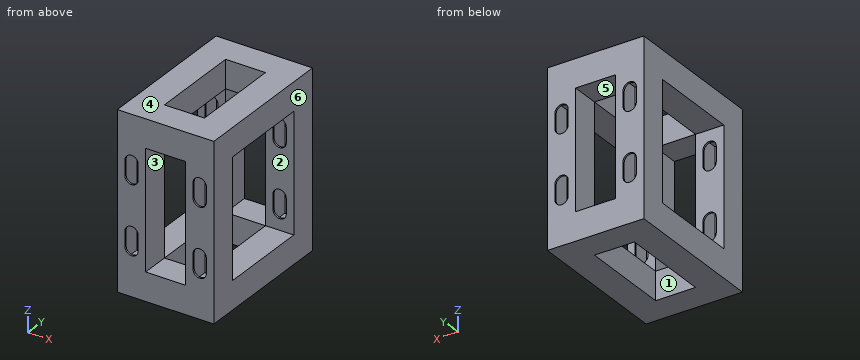
```python
from build123d import *

# Parameters (mm, degrees)
SKETCH2_W          = 19.05
SKETCH2_H          = 19.05
SKETCH2_W_2        = 16.65
SKETCH2_H_2        = 16.65
CUT_EXTRUDE1_START = -9.525
SKETCH1_3_W        = 26.96
SKETCH1_3_H        = 80
CUT_EXTRUDE1_DEPTH = 19.05
SKETCH4_W          = 19.05
SKETCH4_H          = 19.05
SKETCH4_W_2        = 16.65
SKETCH4_H_2        = 16.65


with BuildPart() as part:
    # Sweep1: sweep along a path in Sketch1
    with BuildLine(Plane(origin=(0, 0, 0), x_dir=(1, 0, 0), z_dir=(0, 1, 0))) as sweep1_path:
        Line((13.48, 40), (-13.48, 40))
        Line((-13.48, 40), (-13.48, -40))
        Line((-13.48, -40), (13.48, -40))
        Line((13.48, -40), (13.48, 40))
    # Sketch2 → Sweep1 (sweep)
    with BuildSketch(Plane.XY):
        with Locations((-23.005, 0)):
            Rectangle(SKETCH2_W, SKETCH2_H)
        with Locations((-23.005, 0)):
            Rectangle(SKETCH2_W_2, SKETCH2_H_2, mode=Mode.SUBTRACT)
    sweep(path=sweep1_path.line, transition=Transition.RIGHT)

    # Sketch1<3> → Cut-Extrude1 (cut)
    with BuildSketch(Plane(origin=(0, 0, 0), x_dir=(1, 0, 0), z_dir=(0, 1, 0)).offset(CUT_EXTRUDE1_START)):
        Rectangle(SKETCH1_3_W, SKETCH1_3_H)
        with BuildLine():
            Line((-18.480970389, 27.980970389), (-18.480970389, 17.980970389))
            ThreePointArc((-18.480970389, 17.980970389), (-22.980970389, 13.480970389), (-27.480970389, 17.980970389))
            Line((-27.480970389, 17.980970389), (-27.480970389, 27.980970389))
            ThreePointArc((-27.480970389, 27.980970389), (-22.980970389, 32.480970389), (-18.480970389, 27.980970389))
        make_face()
        with BuildLine():
            Line((-18.480970389, -17.980970389), (-18.480970389, -27.980970389))
            ThreePointArc((-18.480970389, -27.980970389), (-22.980970389, -32.480970389), (-27.480970389, -27.980970389))
            Line((-27.480970389, -27.980970389), (-27.480970389, -17.980970389))
            ThreePointArc((-27.480970389, -17.980970389), (-22.980970389, -13.480970389), (-18.480970389, -17.980970389))
        make_face()
        with BuildLine():
            Line((27.480970389, 27.980970389), (27.480970389, 17.980970389))
            ThreePointArc((27.480970389, 17.980970389), (22.980970389, 13.480970389), (18.480970389, 17.980970389))
            Line((18.480970389, 17.980970389), (18.480970389, 27.980970389))
            ThreePointArc((18.480970389, 27.980970389), (22.980970389, 32.480970389), (27.480970389, 27.980970389))
        make_face()
        with BuildLine():
            Line((18.480970389, -27.980970389), (18.480970389, -17.980970389))
            ThreePointArc((18.480970389, -17.980970389), (22.980970389, -13.480970389), (27.480970389, -17.980970389))
            Line((27.480970389, -17.980970389), (27.480970389, -27.980970389))
            ThreePointArc((27.480970389, -27.980970389), (22.980970389, -32.480970389), (18.480970389, -27.980970389))
        make_face()
    extrude(amount=CUT_EXTRUDE1_DEPTH, mode=Mode.SUBTRACT)

    # Sweep2: sweep along a path in Sketch3
    with BuildLine(Plane(origin=(0, 0, 40), x_dir=(-1, 0, 0), z_dir=(0, 0, -1))) as sweep2_path:
        Line((13.48, 40.475), (13.48, 9.525))
        Line((13.48, 9.525), (-13.48, 9.525))
        Line((-13.48, 9.525), (-13.48, 40.475))
    # Sketch4 → Sweep2 (sweep)
    with BuildSketch(Plane(origin=(0, 9.525, 0), x_dir=(1, 0, 0), z_dir=(0, 1, 0))):
        with Locations((-23.005, -49.525)):
            Rectangle(SKETCH4_W, SKETCH4_H)
        with Locations((-23.005, -49.525)):
            Rectangle(SKETCH4_W_2, SKETCH4_H_2, mode=Mode.SUBTRACT)
    sweep2 = sweep(path=sweep2_path.line, transition=Transition.RIGHT)

    # Mirror1: Sweep2 across plane
    add(sweep2.mirror(Plane.XY))

    # Mirror3: part across plane


with BuildPart() as part_1:
    add(part.part)
    add(part.part.mirror(Plane.ZX.offset(40.475)))


solid = part_1.part
```
Geometry: final body of the model. Coordinates: model frame, mm. Face numbers are marked on the shaded views. A direction names the side the tool comes from. Round coordinates to 2 decimals unless told otherwise and drop trailing zeros. Write each loop counter-clockwise with the first axis right and the second up, starting at its lowest first coordinate (ties: lowest second). Pieces come first, ordered by that corner, then holes. Notation, with made-up numbers: (60.5, 2) -> (114.5, 2) arc R24 cw to (114.5, 16) -> close; hole circle Ø5 at (-5.5, -17). An arc over 180 degrees is marked (long way). Return JSON: item names as keys, results as strings.
Q1. Section C-C on z = 43. Return the cut outline in (x, y) (3 decimals).
From the geometry:
{"outline": "(-32.53, -9.525) -> (32.53, -9.525) -> (32.53, 90.475) -> (-32.53, 90.475) -> close; hole (-31.33, -8.325) -> (31.33, -8.325) -> (31.33, 8.325) -> (-31.33, 8.325) -> close; hole (-31.33, 9.525) -> (-14.68, 9.525) -> (-14.68, 71.425) -> (-31.33, 71.425) -> close; hole (-31.33, 72.625) -> (31.33, 72.625) -> (31.33, 89.275) -> (-31.33, 89.275) -> close; hole (-13.48, 9.525) -> (13.48, 9.525) -> (13.48, 71.425) -> (-13.48, 71.425) -> close; hole (14.68, 9.525) -> (31.33, 9.525) -> (31.33, 71.425) -> (14.68, 71.425) -> close"}
Q2. Section D-D on y = 79. Return the cut outline in (x, z), and give its area (3 significant figures).
From the geometry:
{"outline": "(-32.53, -59.05) -> (32.53, -59.05) -> (32.53, 59.05) -> (-32.53, 59.05) -> close; hole (-31.33, -57.85) -> (31.33, -57.85) -> (31.33, -41.2) -> (-31.33, -41.2) -> close; hole (-31.33, -40) -> (-14.68, -40) -> (-14.68, 40) -> (-31.33, 40) -> close; hole (-31.33, 41.2) -> (31.33, 41.2) -> (31.33, 57.85) -> (-31.33, 57.85) -> close; hole (-13.48, -40) -> (13.48, -40) -> (13.48, 40) -> (-13.48, 40) -> close; hole (14.68, -40) -> (31.33, -40) -> (31.33, 40) -> (14.68, 40) -> close", "area": "776 mm2"}
Q3. Section A-A on z = -38. Give the number of separate pieces and of enclosed holes in the cut face, and give its area (3 significant figures).
From the geometry:
{"separate pieces": "4", "enclosed holes": "4", "area": "343 mm2"}
Q4. Set-up query: the marked faces 1, 2 and 3. Return all of +Z, -Z, +X, -X, +Y, -Y with unobstructed straight access to the full face (end or side cutting, diameter ignored); none if empty.
From the geometry:
{"face 1": "+Z, -Z", "face 2": "+X, -X", "face 3": "+Y, -Y"}
Q5. First-contact query: pin 1 Ø5 at (x, z) = (-11.5, -20.5) entering from +Y (3 decimals). Flat tip, straight axial feed; report the tip coordinate or a pass-through.
From the geometry:
{"pin 1": "y = 90.475"}
Q6. Ray query, line 1 (Z direction, x = 25, y = -4.5); line 2 (Y direction, x = -10, z = -47) (3 decimals); line 3 (X direction, y = 45, z = -44). Return the intervals inside material, ascending.
From the geometry:
{"line 1": "-59.05 to -57.85, -41.2 to -40, 40 to 41.2, 57.85 to 59.05", "line 2": "-9.525 to -8.325, 8.325 to 9.525, 71.425 to 72.625, 89.275 to 90.475", "line 3": "-32.53 to -31.33, -14.68 to -13.48, 13.48 to 14.68, 31.33 to 32.53"}
Q7. Mould query, pull axis X, two halves, no side actions, for the marked faces 4, 5 and 6. Classes: +X half, -X half, draft (parallel to the pull), parting line (faces both ways), or undercut.
From the geometry:
{"face 4": "draft", "face 5": "undercut", "face 6": "+X half"}
